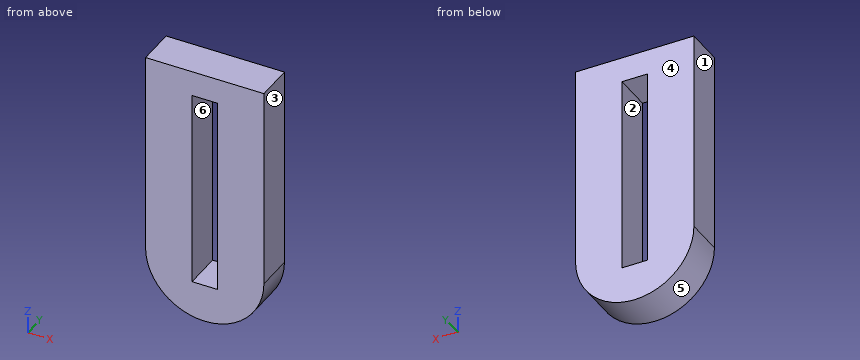
```python
from build123d import *

# Parameters (mm, degrees)
SKETCH1_W           = 12.7
SKETCH1_H           = 99.441
BOSS_EXTRUDE1_DEPTH = 19.05


with BuildPart() as part:
    # Sketch1 → Boss-Extrude1 (new body)
    with BuildSketch(Plane(origin=(0, 0, 0), x_dir=(1, 0, 0), z_dir=(0, 1, 0))):
        with BuildLine():
            Line((-59.182, 0), (0, 0))
            Line((0, 0), (0, 101.6))
            ThreePointArc((0, 101.6), (-29.591, 131.191), (-59.182, 101.6))
            Line((-59.182, 101.6), (-59.182, 0))
        make_face()
        with Locations((-29.591, 62.4205)):
            Rectangle(SKETCH1_W, SKETCH1_H, mode=Mode.SUBTRACT)
    extrude(amount=BOSS_EXTRUDE1_DEPTH)


solid = part.part
```
Geometry check sheet. Reference: the model listing, model coordinates, mm. Face numbers are marked on the shaded views. A direction names the side the tool comes from. Coordinates: 2 decimals unless noted, no trailing zeros. Loops run counter-clockwise (first coordinate to the right, second up) from the corner with the lowest first, then second, coordinate; pieces in that order, holes last. Notation, with made-up numbers: (19.5, 81) - (51.5, 81) arc R6 cw to (51.5, 92) - close; hole circle Ø8 at (2.5, 31.25). An arc over 180 degrees is marked (long way). One line per item, written item: value. Start each with the question number.
(1) Cross-section at A-A on z = -33. Enter the section's corners in (x, y), plus the area to 3 significant figures.
(2) Material ranges on line 1 (X direction, y = 2, z = -72); line 2 (X direction, y = 10, z = -103.5); line 3 (Z direction, x = -33.5, y = 15.25), recorded low to high. Write a range as [from, to].
(3) Mould release check, pull along X, two halves, no side actions. Record for the marked faces 1, 2, 3 and 4: released by +X, released by -X, zero draft, split by the parting line, or undercut.
(4) Cross-section at D-D on z = -118.5. Enter the section's corners in (x, y), plus the area to 3 significant figures.
(5) Depth check by flat-ended pin: P1, Ø2, axis at x = -18, y = 11, coming from the -Z side; P2, Ø10, axis at x = -28, y = 7.5, coming from the -Z side; P3, Ø4, axis at x = -32, z = -49.5, coming from the -Y side. Enter the tip coordinate at first touch or a pass-through.
(6) Tool access check on the marked faces 5 and 6. Record the directions out of +Z, -Z, +X, -X, +Y, -Y that give a thin tool (end or side, any length) a straight path to the whole face; none if there is none.
(7) Cross-section at B-B on y = 1.5. Enter the section's corners in (x, z), plus the area to 3 significant figures.
(8) Cross-section at C-C on x = -13. Enter the section's corners in (y, z).
Results below:
1. outline: (-59.18, 0) - (-35.94, 0) - (-35.94, 19.05) - (-59.18, 19.05) - close; (-23.24, 0) - (0, 0) - (0, 19.05) - (-23.24, 19.05) - close
1. area: 885 mm2
2. line 1: x = [-59.18, -35.94], [-23.24, 0]
2. line 2: x = [-59.12, -35.94], [-23.24, -0.06]
2. line 3: z = [-130.93, -112.14], [-12.7, 0]
3. face 1: released by -X
3. face 2: undercut
3. face 3: released by +X
3. face 4: zero draft
4. outline: (-53.88, 0) - (-5.3, 0) - (-5.3, 19.05) - (-53.88, 19.05) - close
4. area: 925 mm2
5. P1: stops at z = -129.23
5. P2: stops at z = -131.19
5. P3: passes through
6. face 5: -Z, +Y, -Y
6. face 6: +Y, -Y
7. outline: (-59.18, -101.6) arc R29.59 ccw to (0, -101.6) - (0, 0) - (-59.18, 0) - close; hole (-35.94, -112.14) - (-23.24, -112.14) - (-23.24, -12.7) - (-35.94, -12.7) - close
7. area: 6,130 mm2
8. outline: (0, -126.1) - (19.05, -126.1) - (19.05, 0) - (0, 0) - close
